Answer from the drawing. Dimensions are ordinates in mm from the lowest x, y and z of the part. A direction names the side the tool comes from. Round coordinates to 2 decimals unless told otherwise and drop trailing zeros. Write each loop counter-clockwise with the first axis right and the second up, starting at its lowest first coordinate (ties: lowest second). Pieces come first, ordered by that corner, then holes. Notation, with made-up numbers: (-29, -31) - (-24, -31) arc R22 cw to (-24, -20) - close; hole circle Ø1 at (52, 36.5). An arc over 180 degrees is marked (long way). One line per item, written item: value. Start each with the question number.
(1) A cutting plane is placed at A-A, the plane y = 2. Determine the outline of the cut face in (x, z), plus the area to 3 significant figures.
(2) Flat-ended cylindrical pins translate along their axes: pin 1 Ø1 at (x, z) = (20, 70.5) entering from -Y; pin 2 Ø0.9 at (x, y) = (39, 10) entering from -Z. Find the tip coordinate at first contact, or state that the pin passes through.
(3) Find the intervals of material crossed by L1, parallel to Z at x = 48, y = 5; L2, parallel to Z at x = 6.5, y = 6.75; L3, parallel to Y at x = 9, z = 51, in increasing order.
(4) A cutting plane is placed at B-B, the plane x = 42.5. Determine the outline of the cut face in (y, z).
(5) A cutting plane is placed at C-C, the plane x = 6.5. Determine the outline of the cut face in (y, z), plus the area to 3 significant figures.
(6) For the marked faces 4, 5 and 6, determine the directions among +Z, -Z, +X, -X, +Y, -Y from which every point of the face is accessible in a straight line to the end or side of a thin tool.
(7) A cutting plane is placed at D-D, the plane z = 60.5. Determine the outline of the cut face in (x, y), plus the area to 3 significant figures.
(8) The mould has two halves that part along X. Classify the marked faces 1, 2 and 3: +X half, -X half, draft (parallel to the pull), parting line (faces both ways), or undercut.
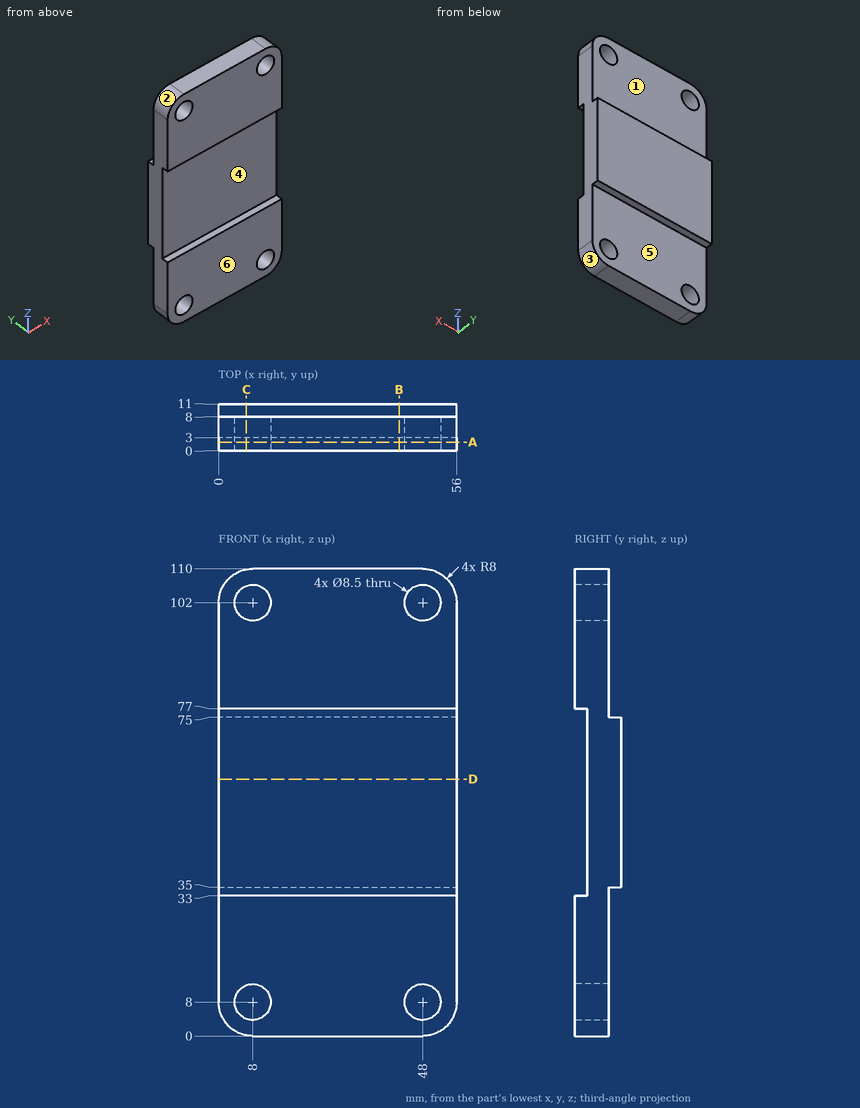
Here are the results:
1. outline: (0, 8) arc R8 ccw to (8, 0) - (48, 0) arc R8 ccw to (56, 8) - (56, 33) - (0, 33) - close; (0, 77) - (56, 77) - (56, 102) arc R8 ccw to (48, 110) - (8, 110) arc R8 ccw to (0, 102) - close; hole circle Ø8.5 at (8, 8); hole circle Ø8.5 at (8, 102); hole circle Ø8.5 at (48, 8); hole circle Ø8.5 at (48, 102)
1. area: 3,410 mm²
2. pin 1: y = 3
2. pin 2: z = 35
3. L1: 0 to 3.75, 12.25 to 97.75, 106.25 to 110
3. L2: 0.14 to 4.02, 11.98 to 98.02, 105.98 to 109.86
3. L3: 3 to 11
4. outline: (0, 0) - (8, 0) - (8, 35) - (11, 35) - (11, 75) - (8, 75) - (8, 110) - (0, 110) - (0, 77) - (3, 77) - (3, 33) - (0, 33) - close
5. outline: (0, 0.14) - (8, 0.14) - (8, 4.02) - (0, 4.02) - close; (0, 11.98) - (8, 11.98) - (8, 35) - (11, 35) - (11, 75) - (8, 75) - (8, 98.02) - (0, 98.02) - (0, 77) - (3, 77) - (3, 33) - (0, 33) - close; (0, 105.98) - (8, 105.98) - (8, 109.86) - (0, 109.86) - close
5. area: 738 mm²
6. face 4: +X, -X, -Y
6. face 5: -Z, +X, -X, +Y
6. face 6: +Z, -Z, +X, -X, -Y
7. outline: (0, 3) - (56, 3) - (56, 11) - (0, 11) - close
7. area: 448 mm²
8. face 1: draft
8. face 2: -X half
8. face 3: +X half
